```python
from build123d import *

# Parameters (mm, degrees)
SKETCH1_W           = 48
SKETCH1_H           = 27
BOSS_EXTRUDE1_DEPTH = 20
SKETCH2_W           = 22
SKETCH2_H           = 15
CUT_EXTRUDE1_DEPTH  = 108.682186993
SKETCH11_R          = 3.25
CUT_EXTRUDE2_DEPTH  = 110.846383385
CHAMFER2_SIZE       = 1
CHAMFER1_SIZE       = 1


with BuildPart() as part:
    # Sketch1 → Boss-Extrude1 (new body)
    with BuildSketch(Plane.XZ.offset(-9.508889291)):
        with Locations((-78.305686037, 13.5)):
            Rectangle(SKETCH1_W, SKETCH1_H)
    extrude(amount=-BOSS_EXTRUDE1_DEPTH)

    # Sketch2 → Cut-Extrude1 (cut, through all)
    with BuildSketch(Plane.XZ.offset(-9.508889291)):
        with Locations((-78.305686037, 13.5)):
            Rectangle(SKETCH2_W, SKETCH2_H)
    extrude(amount=-CUT_EXTRUDE1_DEPTH, mode=Mode.SUBTRACT)

    # Sketch11 → Cut-Extrude2 (cut, through all)
    with BuildSketch(Plane(origin=(0, 0, 0), x_dir=(-1, 0, 0), z_dir=(0, 0, -1))):
        with Locations((94.305686037, 19.508889291)):
            Circle(SKETCH11_R)
        with Locations((62.305686037, 19.508889291)):
            Circle(SKETCH11_R)
    extrude(amount=-CUT_EXTRUDE2_DEPTH, mode=Mode.SUBTRACT)

    # Chamfer2
    chamfer2_edges = [part.edges().sort_by_distance(p)[0] for p in [
        (-89.305686037, 19.508889291, 21),
        (-67.305686037, 19.508889291, 21),
        (-67.305686037, 19.508889291, 6),
        (-89.305686037, 19.508889291, 6),
    ]]
    chamfer(chamfer2_edges, length=CHAMFER2_SIZE)

    # Chamfer1
    chamfer1_edges = [part.edges().sort_by_distance(p)[0] for p in [
        (-54.305686037, 29.508889291, 13.5),
        (-78.305686037, 29.508889291, 27),
        (-91.055686037, 19.508889291, 27),
        (-91.055686037, 19.508889291, 0),
        (-59.055686037, 19.508889291, 27),
        (-59.055686037, 19.508889291, 0),
        (-78.305686037, 9.508889291, 6),
        (-78.305686037, 29.508889291, 6),
        (-89.305686037, 9.508889291, 13.5),
        (-102.305686037, 29.508889291, 13.5),
        (-89.305686037, 29.508889291, 13.5),
        (-67.305686037, 9.508889291, 13.5),
        (-67.305686037, 29.508889291, 13.5),
        (-78.305686037, 9.508889291, 21),
        (-78.305686037, 29.508889291, 21),
        (-78.305686037, 9.508889291, 27),
        (-88.805686037, 9.508889291, 6.5),
        (-88.805686037, 29.508889291, 6.5),
        (-67.805686037, 9.508889291, 6.5),
        (-67.805686037, 29.508889291, 6.5),
        (-67.805686037, 9.508889291, 20.5),
        (-67.805686037, 29.508889291, 20.5),
        (-88.805686037, 9.508889291, 20.5),
        (-54.305686037, 9.508889291, 13.5),
        (-88.805686037, 29.508889291, 20.5),
        (-78.305686037, 9.508889291, 0),
        (-102.305686037, 9.508889291, 13.5),
        (-78.305686037, 29.508889291, 0),
        (-102.305686037, 19.508889291, 27),
        (-54.305686037, 19.508889291, 27),
        (-54.305686037, 19.508889291, 0),
        (-102.305686037, 19.508889291, 0),
    ]]
    chamfer(chamfer1_edges, length=CHAMFER1_SIZE)


solid = part.part
```
Could you check a few things on this model? Use its own coordinates, in mm. A direction names the side the tool comes from. Round coordinates to 2 decimals unless told otherwise and drop trailing zeros. Write each loop counter-clockwise with the first axis right and the second up, starting at its lowest first coordinate (ties: lowest second). Pieces come first, ordered by that corner, then holes. Notation, with made-up numbers: M 55,24.5 L 68,24.5 A24 ccw 68,56.5 Z; hole C -32.75,-32.75 d2. An arc over 180 degrees is marked long. Answer in a Markdown table with one row per item. Add a question column.
Q1. On a 3-axis mill with a long thin cutter (end or side, diameter ignored), from which of +Z, -Z, +X, -X, +Y, -Y can I reach the whole of each face in a straight line? I mean faces 1 (the flat face through (-67.436, 29.016, 20.847)), 2 (the flat face through (-78, 19, 6)), 3 (the flat face through (-78.45, 10.02, 5.51)). Say none if no direction works.
Q2. Will this pin go through, and if not, where does the flat tip stop? pin 1 Ø4 at (x, y) = (-62.31, 19.51) entering from -Z.
Q3. If I drill on line 1 (X direction, y = 19.75, z = 7.5); line 2 (X direction, y = 23.75, z = 8.25); line 3 (Z direction, x = -81.5, y = 25), over which ranges is the centre line in solid material (lowest first)? Write a range as from..to.
Q4. Imagine slicing it at A-A (x = -83.5). Please give me the cut outline in (y, z), then the cut area to 3 significant figures.
Q5. Imagine slicing it at C-C (z = 3.75). Please give me the cut outline in (x, y).
Q6. Imagine slicing it at B-B (y = 24.75). Please give me the cut outline in (x, z).
Q7. Imagine slicing it at D-D (z = 19). Please give me the cut outline in (x, y), then the cut area to 3 significant figures.
Values:
| question | item | result |
|---|---|---|
| 1 | face 1 | +Y |
| 1 | face 2 | +Y, -Y |
| 1 | face 3 | -Y |
| 2 | pin 1 | through |
| 3 | line 1 | -102.31..-97.55, -91.06..-89.31, -67.31..-65.55, -59.06..-54.31 |
| 3 | line 2 | -102.31..-89.31, -67.31..-54.31 |
| 3 | line 3 | 0..6, 21..27 |
| 4 | outline | M 9.51,1 L 10.51,0 L 28.51,0 L 29.51,1 L 29.51,5 L 28.51,6 L 10.51,6 L 9.51,5 Z; M 9.51,22 L 10.51,21 L 28.51,21 L 29.51,22 L 29.51,26 L 28.51,27 L 10.51,27 L 9.51,26 Z |
| 4 | area | 236 mm^2 |
| 5 | outline | M -102.31,10.51 L -101.31,9.51 L -55.31,9.51 L -54.31,10.51 L -54.31,28.51 L -55.31,29.51 L -101.31,29.51 L -102.31,28.51 Z; hole C -94.31,19.51 d6.5; hole C -62.31,19.51 d6.5 |
| 6 | outline | M -102.31,1 L -101.31,0 L -55.31,0 L -54.31,1 L -54.31,26 L -55.31,27 L -101.31,27 L -102.31,26 Z; hole M -89.31,7 L -88.31,6 L -68.31,6 L -67.31,7 L -67.31,20 L -68.31,21 L -88.31,21 L -89.31,20 Z |
| 7 | outline | M -102.31,10.51 L -101.31,9.51 L -90.31,9.51 L -89.31,10.51 L -89.31,28.51 L -90.31,29.51 L -101.31,29.51 L -102.31,28.51 Z; M -67.31,10.51 L -66.31,9.51 L -55.31,9.51 L -54.31,10.51 L -54.31,28.51 L -55.31,29.51 L -66.31,29.51 L -67.31,28.51 Z; hole C -94.31,19.51 d6.5; hole C -62.31,19.51 d6.5 |
| 7 | area | 450 mm^2 |
